Can you work these out from the model? Positions are in its coordinate system, mm. Coordinates: 2 decimals unless noted, no trailing zeros. Return JSON: item names as keys, results as strings. Group by question number.
1) Imagine slicing it at A-A (y = 18). Give the number of separate pieces and of enclosed holes in the cut face, and give its area (3 significant figures).
2) For pin 1 Ø2 at (x, z) = (46, 173) entering from +Y; pin 2 Ø3.5 at (x, z) = (92, 303.5) entering from +Y; pin 3 Ø1.6 at (x, z) = (30.5, 66.5) entering from -Y, each with a flat end and sliding along its axis, tell me the tip position at first contact or that it passes through.
3) If I drill on line 1 along Z through (x, y) = (28, 2); line 2 along Z through (x, y) = (53, 4.75); line 3 along X through (y, z) = (3.8, 179), over which ranges is the centre line in solid material (lowest first)?
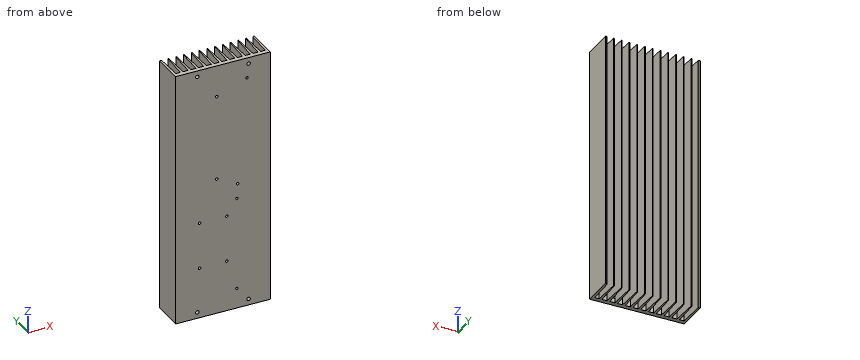
```python
from build123d import *

# Parameters (mm, degrees)
EXTRUDE_1_DEPTH       = 330
EXTRUDE_3_DEPTH       = 330
PATTERN_CURVE_1_COUNT = 11
PATTERN_CURVE_1_PITCH = 10
SKETCH_3_R            = 2.25
CUT_EXTRUDE_1_DEPTH   = 6
SKETCH_4_R            = 1.6
CUT_EXTRUDE_2_DEPTH   = 6


with BuildPart() as part:
    # Эскиз1 → Вытянуть1 (new body)
    with BuildSketch(Plane.XY):
        with BuildLine():
            Line((0, 40), (1.528979332, 40))
            ThreePointArc((1.528979332, 40), (2.225614441, 39.717425624), (2.528547087, 39.029399052))
            Line((2.528547087, 39.029399052), (3.5, 6))
            Line((3.5, 6), (118.5, 6))
            Line((118.5, 6), (119.471452913, 39.029399052))
            ThreePointArc((119.471452913, 39.029399052), (119.774385559, 39.717425624), (120.471020668, 40))
            Line((120.471020668, 40), (122, 40))
            Line((122, 40), (122, 0))
            Line((122, 0), (0, 0))
            Line((0, 0), (0, 40))
        make_face()
    extrude(amount=EXTRUDE_1_DEPTH)

    # Эскиз2 → Вытянуть3 (add)
    with BuildSketch(Plane.XY.offset(330)):
        with BuildLine():
            Line((10.5, 39.5), (9.25, 6))
            Line((9.25, 6), (12.75, 6))
            Line((12.75, 6), (11.5, 39.5))
            ThreePointArc((11.5, 39.5), (11, 40), (10.5, 39.5))
        make_face()
    extrude_3 = extrude(amount=-EXTRUDE_3_DEPTH)

    # Кривая1: Вытянуть3 ×11
    with Locations(*[(i * PATTERN_CURVE_1_PITCH, 0, 0) for i in range(1, PATTERN_CURVE_1_COUNT)]):
        add(extrude_3)

    # Эскиз3 → Вырез-Вытянуть1 (cut)
    with BuildSketch(Plane.XZ):
        with Locations((28, 322)):
            Circle(SKETCH_3_R)
        with Locations((94, 322)):
            Circle(SKETCH_3_R)
        with Locations(Location((94, 8, 0), (0, 0, 236.251011404))):
            Circle(SKETCH_3_R)
        with Locations(Location((28, 8, 0), (0, 0, 56.251011404))):
            Circle(SKETCH_3_R)
    extrude(amount=-CUT_EXTRUDE_1_DEPTH, mode=Mode.SUBTRACT)

    # Эскиз4 → Вырез-Вытянуть2 (cut)
    with BuildSketch(Plane(origin=(147.933613103, 0, 237.946321054), x_dir=(-1, 0, 0), z_dir=(0, -1, 0))):
        with Locations(Location((94.933613103, -51.053678946, 0), (0, 0, 180))):
            Circle(SKETCH_4_R)
        with Locations(Location((116.933613103, 111.946321054, 0), (0, 0, 180))):
            Circle(SKETCH_4_R)
        with Locations(Location((68.933613103, 211.946321054, 0), (0, 0, 180))):
            Circle(SKETCH_4_R)
        with Locations(Location((68.933613103, 91.946321054, 0), (0, 0, 180))):
            Circle(SKETCH_4_R)
        with Locations(Location((81.933613103, 111.946321054, 0), (0, 0, 180))):
            Circle(SKETCH_4_R)
        with Locations(Location((116.933613103, 171.946321054, 0), (0, 0, 180))):
            Circle(SKETCH_4_R)
        with Locations(Location((81.933613103, 171.946321054, 0), (0, 0, 180))):
            Circle(SKETCH_4_R)
        with Locations(Location((94.933613103, 58.946321054, 0), (0, 0, 180))):
            Circle(SKETCH_4_R)
        with Locations(Location((55.933613103, -65.553678946, 0), (0, 0, 180))):
            Circle(SKETCH_4_R)
        with Locations(Location((67.933613103, 72.446321054, 0), (0, 0, 180))):
            Circle(SKETCH_4_R)
    extrude(amount=-CUT_EXTRUDE_2_DEPTH, mode=Mode.SUBTRACT)


solid = part.part
```
Calculated:
{
 "1": {"separate pieces": "13", "enclosed holes": "0", "area": "11,500 mm2"},
 "2": {"pin 1": "y = 6", "pin 2": "y = 40", "pin 3": "y = 6"},
 "3": {"line 1": "0 to 5.75, 10.25 to 319.75, 324.25 to 330", "line 2": "0 to 177.4, 180.6 to 287.4, 290.6 to 330", "line 3": "0 to 51.4, 54.6 to 122"}
}
